Autodesk Inventor part; units mm, degrees
ref_plane "YZ Plane" through (0, 0, 0) normal (1, 0, 0) x (0, 1, 0)
ref_plane "XZ Plane" through (0, 0, 0) normal (0, 1, 0) x (-1, 0, 0)
ref_plane "XY Plane" through (0, 0, 0) normal (0, 0, 1) x (1, 0, 0)
sketch "Sketch2" plane through (0, 0, 0) normal (0, 1, 0) x (-1, 0, 0)
  line L0 (0, 0) -> (67.8, 0)
  line L1 (67.8, 0) -> (67.8, -19.2)
  line L2 (67.8, -19.2) -> (42.8, -19.2)
  line L3 (42.8, -19.2) -> (42.8, -16.2)
  line L4 (42.8, -16.2) -> (65, -16.2)
  line L5 (65, -16.2) -> (65, -8)
  line L6 (65, -8) -> (2.8, -8)
  line L7 (2.8, -8) -> (2.8, -16.2)
  line L8 (2.8, -16.2) -> (25, -16.2)
  line L9 (25, -16.2) -> (25, -19.2)
  line L10 (25, -19.2) -> (0, -19.2)
  line L11 (0, -19.2) -> (0, 0)
  dimension "d2" = 62.2
  dimension "d3" = 2.8
  dimension "d4" = 2.8
  dimension "d5" = 3
  dimension "d6" = 25
  dimension "d7" = 25
  dimension "d8" = 8
  dimension "d9" = 8.2
extrude "Extrusion1" add sketch "Sketch2" along normal blind 10
sketch "Sketch3" plane through (0, 0, 0) normal (0, -1, 0) x (1, 0, 0)
  line L0 (-2.8, -8) -> (-65, -8)
  line L1 (-42.8, -8) -> (-65, -8)
  line L2 (-65, -8) -> (-65, -16.2)
  line L3 (-65, -16.2) -> (-42.8, -16.2)
  line L4 (-42.8, -16.2) -> (-42.8, -8)
  line L5 (-42.8, -19.2) -> (-42.8, -16.2)
  line L6 (-42.8, -16.2) -> (-65, -16.2)
  line L7 (-25, -16.2) -> (-2.8, -16.2)
  line L8 (-2.8, -16.2) -> (-2.8, -8)
  line L9 (-2.8, -8) -> (-25, -8)
  line L10 (-25, -8) -> (-25, -16.2)
  line L11 (-65, -8) -> (-65, -16.2)
  point P0 (0, 0)
extrude "Extrusion2" add sketch "Sketch3" against normal blind 5
sketch "Sketch7" plane through (0, 10, 0) normal (0, 1, 0) x (1, 0, 0)
  line L0 (0, 10) -> (0, 0)
  line L1 (0, 0) -> (-67.8, 0)
  line L2 (-67.8, 0) -> (-67.8, 19.2)
  line L3 (0, 10) -> (0, 19.2)
  line L4 (0, 19.2) -> (-2.8, 19.2)
  line L5 (-2.8, 19.2) -> (-2.8, 8)
  line L6 (-2.8, 8) -> (-65, 8)
  line L7 (-65, 8) -> (-65, 19.2)
  line L8 (-65, 19.2) -> (-67.8, 19.2)
  line L9 (-67.8, 19.2) -> (-67.8, 0)
  line L10 (0, 19.2) -> (-25, 19.2)
  line L11 (-2.8, 8) -> (-65, 8)
  line L12 (-65, 8) -> (-65, 16.2)
  line L13 (-2.8, 16.2) -> (-2.8, 8)
extrude "Extrusion5" add sketch "Sketch7" along normal blind 73
sketch "Sketch10" plane through (0, 83, 0) normal (0, 1, 0) x (1, 0, 0)
  line L0 (-18.9, 0) -> (-48.9, 0)
  line L1 (-48.9, 0) -> (-48.9, 5)
  line L2 (-48.9, 5) -> (-18.9, 5)
  line L3 (-18.9, 5) -> (-18.9, 0)
  line L4 (-2.8, 8) -> (-65, 8)
  line L5 (-67.8, 0) -> (0, 0)
  line L6 (-33.9, 8) -> (-33.9, 19.521) construction
  line L7 (-33.9, 0) -> (-33.9, -9.399) construction
  dimension "d40" = 3
  dimension "d41" = 30
extrude "Extrusion8" cut sketch "Sketch10" against normal blind 40
sketch "Sketch11" plane through (-48.9, 83, -5) normal (0, 0, 1) x (1, 0, 0)
  line L0 (0, 0) -> (1, 0)
  line L1 (1, 0) -> (1, -40)
  line L2 (1, -40) -> (0, -40)
  line L3 (0, -40) -> (0, 0)
  line L4 (29, 0) -> (30, 0)
  line L5 (30, 0) -> (30, -40)
  line L6 (30, -40) -> (29, -40)
  line L7 (29, -40) -> (29, 0)
  line L8 (30, -40) -> (0, -40)
  line L9 (30, 0) -> (30, -40)
  line L10 (0, -40) -> (0, 0)
  line L11 (0, 0) -> (30, 0)
  point P0 (48.9, -83)
  dimension "d44" = 1
  dimension "d45" = 1
extrude "Extrusion9" cut sketch "Sketch11" against normal blind 30 contours L0 L1 L2 L3 | L4 L5 L6 L7
sketch "Sketch13" plane through (-2.8, 5, -8) normal (0, 0, -1) x (-1, 0, 0)
  line L0 (45.1, 78) -> (17.1, 78)
  line L1 (17.1, 78) -> (17.1, 73)
  line L2 (17.1, 73) -> (45.1, 73)
  line L3 (45.1, 73) -> (45.1, 78)
  line L4 (17.1, 78) -> (45.1, 78)
  line L5 (17.1, 78) -> (17.1, 38)
  line L6 (45.1, 38) -> (45.1, 78)
  point P0 (-2.8, -5)
  dimension "d48" = 5
extrude "Extrusion10" add sketch "Sketch13" along normal blind 3
chamfer "Chamfer1" distance 4 angle 45 1 edges at (-33.9, 83, -11)
fillet "Fillet1" radius 5 1 edges at (-33.9, 43, -5)
fillet "Fillet2" radius 2 4 edges at (0, 0, -9.6) (0, 83, -9.6) (-67.8, 0, -9.6) (-67.8, 83, -9.6)
sketch "Sketch16" plane through (-2.8, 5, -8) normal (0, 0, -1) x (-1, 0, 0)
  line L0 (65, 21.0579) -> (48, 21.0579)
  line L1 (48, 21.0579) -> (48, 7.5579)
  line L2 (48, 7.5579) -> (65, 7.5579)
  line L3 (65, 7.5579) -> (65, 21.0579)
  line L4 (24.35, 12) -> (37.85, 12)
  line L5 (37.85, 12) -> (37.85, -5)
  line L6 (37.85, -5) -> (24.35, -5)
  line L7 (24.35, -5) -> (24.35, 12)
  line L8 (40, -5) -> (22.2, -5)
  line L9 (22.2, -5) -> (22.2, 5)
  line L10 (62.2, 5) -> (62.2, 78)
  line L11 (65, -3) -> (65, 76)
  line L12 (-2.8, 21.0579) -> (14.2, 21.0579)
  line L13 (14.2, 21.0579) -> (14.2, 7.5579)
  line L14 (14.2, 7.5579) -> (-2.8, 7.5579)
  line L15 (-2.8, 7.5579) -> (-2.8, 21.0579)
  line L16 (-2.8, -3) -> (-2.8, 76)
  point P0 (-2.8, -5)
  dimension "d80" = 13.5
  dimension "d81" = 17
  dimension "d82" = 13.5
  dimension "d83" = 17
  dimension "d84" = 2.15
  dimension "d138" = 17
extrude "Extrusion15" cut sketch "Sketch16" against normal blind 4
sketch "Sketch8" plane through (-25, 0, -8) normal (0, 0, -1) x (-1, 0, 0)
  circle A0 centre (4.65, 14.5) radius 1.25
  circle A1 centre (13.15, 14.5) radius 1.25
  line L0 (2.15, 17) -> (15.65, 17)
  line L1 (2.15, 0) -> (2.15, 17)
  line L2 (15.65, 17) -> (15.65, 0)
  circle A2 centre (28.3, 23.5579) radius 1.25
  circle A3 centre (28.3, 15.0579) radius 1.25
  line L3 (25.8, 26.0579) -> (40, 26.0579)
  line L4 (25.8, 12.5579) -> (25.8, 26.0579)
  line L5 (40, 12.5579) -> (25.8, 12.5579)
  circle A4 centre (-10.5, 23.5579) radius 1.25
  circle A5 centre (-10.5, 15.0579) radius 1.25
  line L6 (-8, 26.0579) -> (-8, 12.5579)
  line L7 (-8, 12.5579) -> (-25, 12.5579)
  line L8 (-25, 26.0579) -> (-8, 26.0579)
  point P0 (-25, 0)
  dimension "d28" = 2.5
  dimension "d29" = 2.5
  dimension "d87" = 2.5
  dimension "d88" = 2.5
  dimension "d89" = 2.5
  dimension "d90" = 2.5
  dimension "d91" = 2.5
  dimension "d92" = 2.5
  dimension "d93" = 2.5
  dimension "d94" = 2.5
  dimension "d95" = 2.5
  dimension "d96" = 2.5
  dimension "d139" = 2.5
  dimension "d140" = 2.5
  dimension "d141" = 2.5
  dimension "d142" = 2.5
  dimension "d143" = 2.5
  dimension "d144" = 2.5
extrude "Extrusion16" cut sketch "Sketch8" against normal up to surface (8 mm away)
sketch "Sketch15" plane through (-67.8, 0, 0) normal (0, 0, 1) x (1, 0, 0)
  circle A0 centre (53.3, 15.0579) radius 3
  circle A1 centre (53.3, 23.5579) radius 3
  circle A2 centre (38.15, 14.5) radius 3
  circle A3 centre (29.65, 14.5) radius 3
  circle A4 centre (14.5, 15.0579) radius 3
  circle A5 centre (14.5, 23.5579) radius 3
  circle A6 centre (53.3, 15.0579) radius 1.25
  circle A7 centre (53.3, 23.5579) radius 1.25
  circle A8 centre (38.15, 14.5) radius 1.25
  circle A9 centre (29.65, 14.5) radius 1.25
  circle A10 centre (14.5, 15.0579) radius 1.25
  circle A11 centre (14.5, 23.5579) radius 1.25
  point P0 (67.8, 0)
  dimension "d145" = 6
  dimension "d146" = 6
  dimension "d147" = 6
  dimension "d148" = 6
  dimension "d149" = 6
  dimension "d150" = 6
extrude "Extrusion17" cut sketch "Sketch15" against normal blind 3
sketch "Sketch18" plane through (0, 83, 0) normal (0, 1, 0) x (1, 0, 0)
  line L0 (-67.8, 0) -> (-59.8, 0)
  line L1 (-59.8, 0) -> (-59.8, 5)
  line L2 (-59.8, 5) -> (-67.8, 5)
  line L3 (-67.8, 5) -> (-67.8, 0)
  point P0 (0, 0)
  dimension "d116" = 8
  dimension "d117" = 5
extrude "Extrusion19" cut sketch "Sketch18" against normal blind 50
sketch "Sketch21" plane through (-47.9, 83, -5) normal (0, 0, 1) x (1, 0, 0)
  line L0 (28, -35) -> (28, 0)
  line L1 (0, -5) -> (28, -5)
  line L2 (28, -5) -> (28, 5)
  line L3 (28, 5) -> (0, 5)
  line L4 (0, 5) -> (0, -5)
  line L5 (0, 0) -> (0, -35)
  line L6 (0, -5) -> (28, -5)
  point P0 (47.9, -83)
extrude "Extrusion22" add sketch "Sketch21" along normal up to surface (5 mm away)
chamfer "Chamfer2" distance 4 angle 45 1 edges at (-33.9, 88, -5)
chamfer "Chamfer3" distance 4 angle 45 1 edges at (-33.9, 78, -5)
sketch "Sketch19" plane through (0, 83, 0) normal (0, 1, 0) x (1, 0, 0)
  line L0 (-2.8, 19.2) -> (-17.8, 19.2)
  line L1 (-17.8, 19.2) -> (-17.8, 17.2)
  line L2 (-17.8, 17.2) -> (-2.8, 17.2)
  line L3 (-2.8, 17.2) -> (-2.8, 19.2)
  point P0 (0, 0)
  dimension "d120" = 15
  dimension "d151" = 2
sketch "Sketch17" plane through (0, 83, 0) normal (0, 1, 0) x (1, 0, 0)
  line L0 (-65, 17.2) -> (-62.5, 17.2)
  line L1 (-62.5, 17.2) -> (-62.5, 19.2)
  line L2 (-62.5, 19.2) -> (-65, 19.2)
  line L3 (-65, 19.2) -> (-65, 17.2)
  line L4 (-65, 16.2) -> (-42.8, 16.2)
  line L5 (-65, 8) -> (-65, 19.2)
  line L6 (-42.8, 19.2) -> (-65, 19.2)
  point P0 (0, 0)
  dimension "d111" = 2
  dimension "d112" = 2.5
sketch "Sketch20" plane through (0, 2, 0) normal (1, 0, 0) x (0, 0, -1)
  line L0 (19.2, 67) -> (9.5, 67)
  line L1 (9.5, 67) -> (9.5, 12)
  line L2 (9.5, 12) -> (19.2, 12)
  line L3 (19.2, 12) -> (19.2, 67)
  line L4 (19.2, 81) -> (0, 81)
  line L5 (0, -2) -> (19.2, -2)
  line L6 (19.2, 0) -> (19.2, 79)
  line L7 (8, 3) -> (8, 81)
  dimension "d123" = 14
  dimension "d124" = 14
  dimension "d126" = 1.5
ref_plane "Work Plane2" through (-33.9, 2, 0) normal (1, 0, 0) x (0, 0, -1)
extrude "Extrusion25" add sketch "Sketch17" against normal up to next
extrude "Extrusion23" cut sketch "Sketch20" against normal up to surface (5.3 mm away) from surface at -62.5
extrude "Extrusion24" add sketch "Sketch19" against normal blind 20
fillet "Fillet5" radius 2 1 edges at (-17.8, 83, -18.2)
properties part number "ZAPATO ZOWI IZQ2.1"
Model file for the job. Use its own axes, mm. A direction names the side the tool comes from. Round coordinates to 2 decimals unless told otherwise and drop trailing zeros. Order: outer loops, then holes, each group sorted by start corner. A loop starts at its lowest first (then second) coordinate and runs counter-clockwise, first axis right, second up.
(1) Drill centre lines: line 1 (Y direction, x = -14.5, z = -1.2); line 2 (Y direction, x = -3.5, z = -17.25); line 3 (Y direction, x = -53.3, z = -3.55). Where is each one in solid material? Low to high.
(2) 3-axis set-ups, long thin cutter, end or side, ignore diameter. For faces 1 (the face through (-10, 63, -18)), 2 (the face through (-13, 24, -3)), 3 (the face through (-34, 81, -9)), 4 (the face through (-18.9, 63, -4)), 5 (the face through (-40.65, 9, -6)): which of +Z, -Z, +X, -X, +Y, -Y reach the whole face in a straight line?
(3) Band-saw the part on B-B (z = -12). List the corners of the cut face in (x, y).
(4) Pull direction X, two halves, no side cores. Call faces 6 (the face through (-57, 83, -5)), 7 (the face through (-0.6, 0.57, -9.47)), 8 (the face through (-64, 76, -17.2)): released by +X, released by -X, zero draft, split by the parting line, or undercut.
(5) Band-saw the part on A-A (x = -14.5). Give the number of separate pieces and of enclosed holes in the cut face, then the cut area to 3 significant figures.
(6) Band-saw the part on D-D (y = 7). List the corners of the cut face in (x, z), then the cut area to 3 significant figures.
(7) Pin check, flat tips, straight feed: pin 1 (2 mm diameter, centred on x = -22.5, y = 65.5, fed in from +Z); pin 2 (4 mm diameter, centred on x = -14.5, y = 15.06, fed in from -Z); pin 3 (4 mm diameter, centred on x = -50, z = -6.5, fed in from +Y). Stop position of each tip, or through.
Verdict:
1. line 1: y = 0 to 12.06, 18.06 to 20.56, 26.56 to 83
1. line 2: y = 0 to 10, 63 to 83
1. line 3: y = 0 to 13.81, 16.31 to 22.31, 24.81 to 83
2. face 1: -Z, -X
2. face 2: +Z
2. face 3: -Z, +Y
2. face 4: +Z, -Z, +Y
2. face 5: -Z, -Y
3. outline: (-67.8, 2) arc R2 ccw to (-65.8, 0) - (-42.8, 0) - (-42.8, 5) - (-65, 5) - (-65, 14) - (-67.8, 14) - close; (-67.8, 69) - (-65, 69) - (-65, 83) - (-65.8, 83) arc R2 ccw to (-67.8, 81) - close; (-25, 0) - (-2, 0) arc R2 ccw to (0, 2) - (0, 81) arc R2 ccw to (-2, 83) - (-2.8, 83) - (-2.8, 5) - (-25, 5) - close
4. face 6: zero draft
4. face 7: released by +X
4. face 8: undercut
5. separate pieces: 4
5. enclosed holes: 0
5. area: 680 mm2
6. outline: (-67.8, -19.2) - (-42.8, -19.2) - (-42.8, -16.2) - (-65, -16.2) - (-65, -8) - (-40.65, -8) - (-40.65, -4) - (-27.15, -4) - (-27.15, -8) - (-2.8, -8) - (-2.8, -16.2) - (-25, -16.2) - (-25, -19.2) - (0, -19.2) - (0, 0) - (-67.8, 0) - close
6. area: 684 mm2
7. pin 1: stops at z = -5
7. pin 2: stops at z = -4
7. pin 3: stops at y = 83
